Read the model definition and answer for the solid it produces. Units are mm, in the model's axes. Face numbers are marked on the shaded views. A direction names the side the tool comes from. Round coordinates to 2 decimals unless told otherwise and drop trailing zeros. Order: outer loops, then holes, each group sorted by start corner. A loop starts at its lowest first (then second) coordinate and runs counter-clockwise, first axis right, second up. Notation, with made-up numbers: (29.5, 66) - (46.5, 66) arc R21 cw to (46.5, 76) - close; hole circle Ø7 at (10, 52.5). An arc over 180 degrees is marked (long way). Answer as a JSON object with one key per item and string values. Group by question number.
Q1. A cutting plane is placed at C-C on x = 10. Determine the outline of the cut face in (y, z).
Q2. Consider line 1 (Y direction, x = 2.5, z = 5.25); line 2 (X direction, y = 0.65, z = 4.5) (3 decimals); line 3 (X direction, y = 3.35, z = 0.5). Determine where each line is inside the solid, lowest interval first.
Q3. A cutting plane is placed at B-B on z = 0.5. Determine the outline of the cut face in (x, y).
Q4. A cutting plane is placed at A-A on y = 1.8. Determine the outline of the cut face in (x, z), and give its area (3 significant figures).
Q5. A cutting plane is placed at D-D on x = -1.5. Determine the outline of the cut face in (y, z), and give its area (3 significant figures).
Q6. The mould has two halves that part along X. Classify the marked faces 4, 5, 6 and 7: pulls with the +X half, pulls with the -X half, needs draft (parallel to the pull), parting line crosses it, or undercut.
Q7. A tool of negligible diameter and unlimited length cuts with its end or side. For the marked faces 1, 2 and 3, from which of +Z, -Z, +X, -X, +Y, -Y can it reach the whole face along a straight path? Write none if from no direction.
Q8. Given pin 1 Ø3.5 at (x, y) = (9.5, 1.5) entering from +Z; pin 2 Ø2 at (y, z) = (0.5, 5.5) entering from +X (3 decimals); pin 3 Ø0.6 at (y, z) = (0.5, 4.5) entering from -X (3 decimals), each flat-ended and moving along its own axis, determine where each tip first touches the part or whether it passes through.
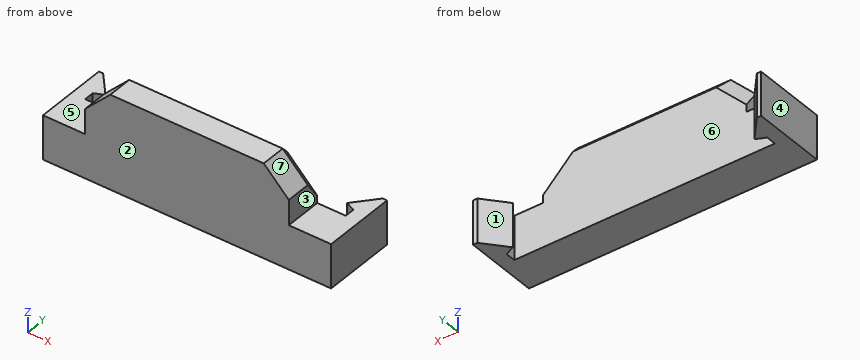
```python
from build123d import *

# Parameters (mm, degrees)
RESSALTO_EXTRUS_O1_DEPTH = 3.5
ESBO_O3_W                = 3.5
ESBO_O3_H                = 5.900568868
CORTE_EXTRUS_O1_DEPTH    = 0.5
ESBO_O4_W                = 3.5
ESBO_O4_H                = 5.900568868
CORTE_EXTRUS_O2_DEPTH    = 0.5
ESBO_O5_W                = 16.25
ESBO_O5_H                = 3
RESSALTO_EXTRUS_O2_DEPTH = 4
CHANFRO1_SIZE            = 2
CHANFRO4_SIZE            = 1


with BuildPart() as part:
    # Esboço2 → Ressalto-extrusão1 (new body)
    with BuildSketch(Plane.XY):
        Polygon((12, 4.400568868), (11.156062048, 4.400568868), (9.648231551, 2.650555385), (10.4, 2.3), (10.4, 1.5), (-10.4, 1.5), (-10.4, 2.3), (-9.648231551, 2.650555385), (-11.156062048, 4.400568868), (-11.996, 4.400568868), (-11.996, -1.5), (12, -1.5), align=None)
    extrude(amount=RESSALTO_EXTRUS_O1_DEPTH)

    # Esboço3 → Corte-extrusão1 (cut)
    with BuildSketch(Plane(origin=(12, 0, 0), x_dir=(0, 0, -1), z_dir=(1, 0, 0))):
        with Locations((-1.75, 1.450284434)):
            Rectangle(ESBO_O3_W, ESBO_O3_H)
    extrude(amount=-CORTE_EXTRUS_O1_DEPTH, mode=Mode.SUBTRACT)

    # Esboço4 → Corte-extrusão2 (cut)
    with BuildSketch(Plane.ZY.offset(11.996)):
        with Locations((1.75, 1.450284434)):
            Rectangle(ESBO_O4_W, ESBO_O4_H)
    extrude(amount=-CORTE_EXTRUS_O2_DEPTH, mode=Mode.SUBTRACT)

    # Esboço5 → Ressalto-extrusão2 (add)
    with BuildSketch(Plane.XY.offset(3.5)):
        Rectangle(ESBO_O5_W, ESBO_O5_H)
    extrude(amount=RESSALTO_EXTRUS_O2_DEPTH)

    # Chanfro1
    chanfro1_edges = [part.edges().sort_by_distance(p)[0] for p in [
        (8.125, 0, 7.5),
        (-8.125, 0, 7.5),
    ]]
    chamfer(chanfro1_edges, length=CHANFRO1_SIZE)

    # Chanfro4
    chanfro4_edges = [part.edges().sort_by_distance(p)[0] for p in [
        (0, 1.5, 7.5),
        (7.125, 1.5, 6.5),
        (-7.125, 1.5, 6.5),
    ]]
    chamfer(chanfro4_edges, length=CHANFRO4_SIZE)


solid = part.part
```
Result set:
{
 "1": {"outline": "(-1.5, 0) - (1.5, 0) - (1.5, 3.5) - (-1.5, 3.5) - close; (2.49, 0) - (3.06, 0) - (3.06, 3.5) - (2.49, 3.5) - close"},
 "2": {"line 1": "y = -1.5 to 1.5", "line 2": "x = -8.125 to 8.125", "line 3": "x = -11.5 to -10.25, 10.25 to 11.5"},
 "3": {"outline": "(-11.5, -1.5) - (11.5, -1.5) - (11.5, 4.4) - (11.16, 4.4) - (9.65, 2.65) - (10.4, 2.3) - (10.4, 1.5) - (-10.4, 1.5) - (-10.4, 2.3) - (-9.65, 2.65) - (-11.16, 4.4) - (-11.5, 4.4) - close"},
 "4": {"outline": "(-11.5, 0) - (-10.4, 0) - (-10.4, 3.5) - (-11.5, 3.5) - close; (10.4, 0) - (11.5, 0) - (11.5, 3.5) - (10.4, 3.5) - close", "area": "7.69 mm²"},
 "5": {"outline": "(-1.5, 0) - (1.5, 0) - (1.5, 6.5) - (0.5, 7.5) - (-1.5, 7.5) - close", "area": "22.0 mm²"},
 "6": {"face 4": "pulls with the -X half", "face 5": "needs draft", "face 6": "undercut", "face 7": "pulls with the +X half"},
 "7": {"face 1": "+Z, -Z, +Y", "face 2": "+Z, -Z, +X, -X, -Y", "face 3": "+Z, +X, +Y, -Y"},
 "8": {"pin 1": "stops at z = 5.56", "pin 2": "stops at x = 8.125", "pin 3": "stops at x = -8.125"}
}
